from build123d import *

# Parameters (mm, degrees)
SKETCH1_W           = 300
SKETCH1_H           = 300
BOSS_EXTRUDE1_DEPTH = 600
SKETCH2_R           = 142.6010694
CUT_EXTRUDE1_DEPTH  = 142.6
REVOLVE1_ANGLE      = 180


with BuildPart() as part:
    # Sketch1 → Boss-Extrude1 (new body)
    with BuildSketch(Plane(origin=(0, 0, 0), x_dir=(1, 0, 0), z_dir=(0, 1, 0))):
        Rectangle(SKETCH1_W, SKETCH1_H)
    extrude(amount=BOSS_EXTRUDE1_DEPTH)

    # Sketch2 → Cut-Extrude1 (cut)
    with BuildSketch(Plane.XZ):
        with Locations(Location((0, 0, 0), (0, 0, 270))):
            Circle(SKETCH2_R)
    extrude(amount=-CUT_EXTRUDE1_DEPTH, mode=Mode.SUBTRACT)

    # Sketch3 → Revolve1 (revolve)
    with BuildSketch(Plane.XZ.offset(-142.6)):
        with BuildLine():
            Line((0, 142.601069387), (0, -142.601069387))
            ThreePointArc((0, -142.601069387), (-142.601069387, 0), (0, 142.601069387))
        make_face()
    revolve(axis=Axis((0, 142.6, 142.601069387), (0, 0, 1)), revolution_arc=REVOLVE1_ANGLE)


solid = part.part
The listing builds one solid part. Answer for the finished solid, in the listing's coordinates (mm). Round coordinates to 2 decimals unless told otherwise and drop trailing zeros. Write each loop counter-clockwise with the first axis right and the second up, starting at its lowest first coordinate (ties: lowest second). Pieces come first, ordered by that corner, then holes. Notation, with made-up numbers: (10, -4) - (63, -4) arc R28 cw to (63, 31) - close; hole circle Ø9 at (-12, 72). An arc over 180 degrees is marked (long way). Use one line per item in the form item = value. Start each with the question number.
Item 1: Determine the mould class of faces 1 (the flat face through (-2, 296, 150)), 2 (the flat face through (150, 296, 2)), 3 (the cylindrical face through (42.833, 70.302, -136.016)) for opening direction X: +X half, -X half, draft (parallel to the pull), parting line (faces both ways), or undercut.
Item 2: Find the intervals of material crossed by line 1 (X direction, y = 110.5, z = 76); line 2 (X direction, y = 38.5, z = 0); line 3 (Z direction, x = 67.5, y = 47.5), in increasing order. Write a range as [from, to].
Item 3: A cutting plane is placed at A-A (z = 0). Write down the section's boundary in (x, y), plus the area to 3 significant figures.
Item 4: Flat-ended cylindrical pins translate along their axes: pin 1 Ø4 at (x, z) = (26, -117.5) entering from -Y; pin 2 Ø4 at (x, z) = (65, 104) entering from -Y. Find the tip coordinate at first contact, or state that the pin passes through.
Item 5: A cutting plane is placed at B-B (x = 0). Write down the section's boundary in (y, z).
The answers:
q1.face_1 = draft
q1.face_2 = +X half
q1.face_3 = undercut
q2.line_1 = [-150, -120.66], [-116.31, 116.31], [120.66, 150]
q2.line_2 = [-150, -142.6], [-97.46, 97.46], [142.6, 150]
q2.line_3 = [-150, -125.61], [-82.07, 82.07], [125.61, 150]
q3.outline = (-150, 0) - (-142.6, 0) - (-142.6, 142.6) arc R142.6 ccw to (142.6, 142.6) - (142.6, 0) - (150, 0) - (150, 600) - (-150, 600) - close
q3.area = 171,000 mm^2
q4.pin_1 = 63.04
q4.pin_2 = 66.57
q5.outline = (0, -150) - (600, -150) - (600, 150) - (0, 150) - (0, 142.6) - (142.6, 142.6) arc R142.6 ccw to (142.6, -142.6) - (0, -142.6) - close
